```python
from build123d import *

# Parameters (mm, degrees)
F0_R     = 38.1
F1_DEPTH = 127
F2_R     = 20.3692597416
F3_DEPTH = 127.001
F5_DEPTH = 127.001


with BuildPart() as f1:
    # F0 (on Top) → F1 (new body)
    with BuildSketch(Plane.XY):
        Circle(F0_R)
    extrude(amount=F1_DEPTH)

    # F2 (on face) → F3 (cut, through all)
    with BuildSketch(Plane.XY.offset(127)):
        Circle(F2_R)
    extrude(amount=-F3_DEPTH, mode=Mode.SUBTRACT)

    # F4 (on face) → F5 (cut, through all)
    with BuildSketch(Plane.XY.offset(127)):
        with BuildLine():
            ThreePointArc((-25.4, 28.3980633142), (-38.1, 0), (-25.4, -28.3980633142))
            Line((-25.4, -28.3980633142), (-25.4, 28.3980633142))
        make_face()
    extrude(amount=-F5_DEPTH, mode=Mode.SUBTRACT)


solid = f1.part
```
The model under review builds one solid part; all positions refer to its coordinate system, in mm. Round coordinates to 2 decimals unless told otherwise and drop trailing zeros. Order: outer loops, then holes, each group sorted by start corner. A loop starts at its lowest first (then second) coordinate and runs counter-clockwise, first axis right, second up. Notation, with made-up numbers: M 87,5.25 L 144,5.25 A30 ccw 144,40.25 Z; hole C 6.25,-35 d8. An arc over 180 degrees is marked long. Use a Markdown table: item, result.
1) Consider section A-A (y = 0). Write out the cut boundary in (x, z), then the cut area to 3 significant figures.
Report:
| item | result |
|---|---|
| outline | M -25.4,0 L -20.37,0 L -20.37,127 L -25.4,127 Z; M 20.37,0 L 38.1,0 L 38.1,127 L 20.37,127 Z |
| area | 2,890 mm^2 |
2) Consider section C-C (z = 49). Write out the cut boundary in (x, y), then the cut area to 3 significant figures.
Report:
| item | result |
|---|---|
| outline | M -25.4,-28.4 A38.1 ccw long -25.4,28.4 Z; hole C 0,0 d40.74 |
| area | 2,760 mm^2 |
3) Insertion check: pin 1 (1 mm diameter, centred on x = 23.5, z = 26, fed in from +Y); pin 2 (10 mm diameter, centred on x = 21.5, z = 29, fed in from -Y); pin 3 (12 mm diameter, centred on x = 2, z = 91.5, fed in from +Y). Each pin has a flat end and moves straight along its axis. Give the tip position at first contact, or say it passes through.
Report:
| item | result |
|---|---|
| pin 1 | y = 30.37 |
| pin 2 | y = -34.34 |
| pin 3 | y = 38.1 |
4) Wall thickness on line 1 along Y through (x, z) = (0, 89.5); line 2 along X through (y, z) = (-11, 102.5); line 3 along Y through (x, z) = (1, 52): over which ranges is each line inside the solid? List them lowest first. Write a range as [from, to].
Report:
| item | result |
|---|---|
| line 1 | [-38.1, -20.37], [20.37, 38.1] |
| line 2 | [-25.4, -17.14], [17.14, 36.48] |
| line 3 | [-38.09, -20.34], [20.34, 38.09] |
5) Consider section B-B (x = 0). Write out the cut boundary in (y, z).
Report:
| item | result |
|---|---|
| outline | M -38.1,0 L -20.37,0 L -20.37,127 L -38.1,127 Z; M 20.37,0 L 38.1,0 L 38.1,127 L 20.37,127 Z |
